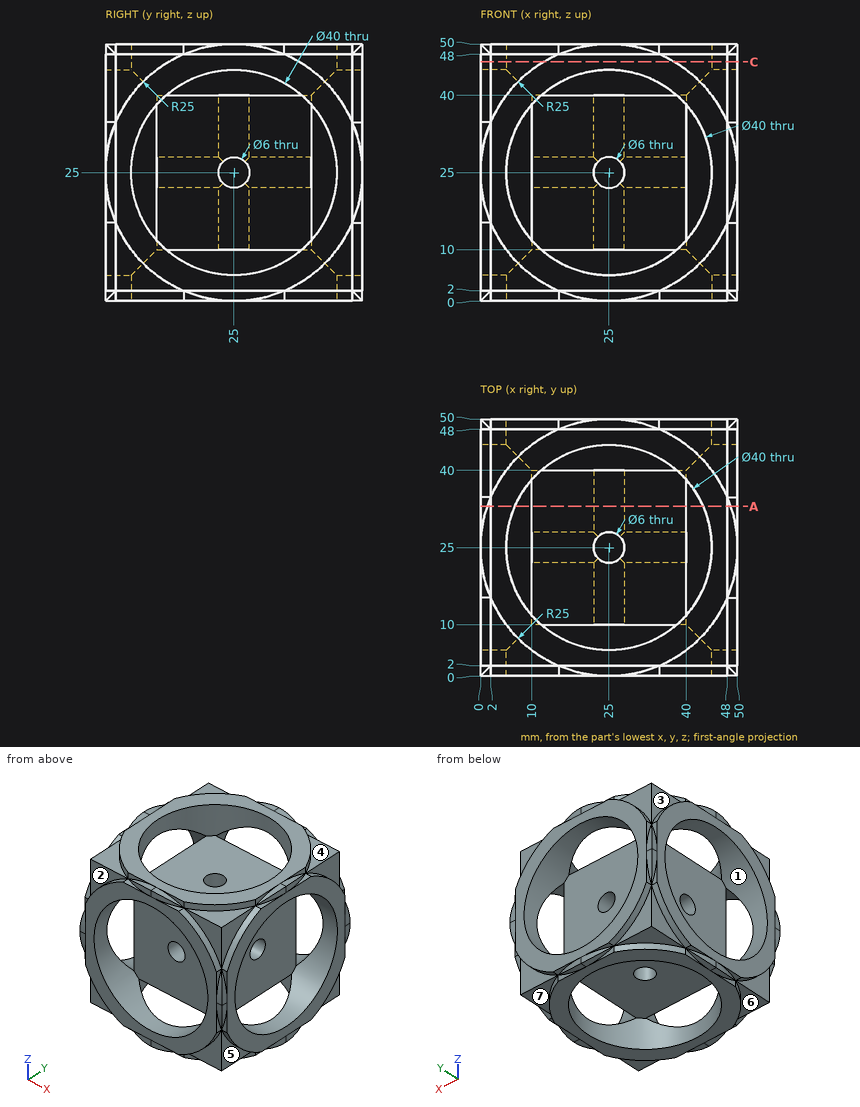
Design review of the part shown in the three views and the two pictorial views. Dimensions are in mm from the part's minimum x, y and z. A direction names the side the tool comes from. Round coordinates to 2 decimals unless told otherwise and drop trailing zeros. Write each loop counter-clockwise with the first axis right and the second up, starting at its lowest first coordinate (ties: lowest second). Pieces come first, ordered by that corner, then holes. Notation, with made-up numbers: (69.25, -9) - (83.25, -9) arc R17 cw to (83.25, 24) - close; hole circle Ø8 at (67, 25.25). An arc over 180 degrees is marked (long way). Write item = value, one per line. Start each with the question number.
1. Consider section C-C on z = 46.5. State the section outline as (x, y) points, plus the area to 3 significant figures.
2. Draft analysis for pull direction Y (two halves, no side actions). For the marked faces 1, 2 and 3, state which applies: released by +Y, released by -Y, zero draft, split by the parting line, or undercut.
3. For the marked faces 4, 5, 6 and 7, list the 3-axis set-ups (+Z, -Z, +X, -X, +Y, -Y) from which the entire face can be reached by the end or side of a thin tool; tool diameter is ignored.
4. Wall thickness on L1, parallel to Z at x = 33, y = 36; L2, parallel to Z at x = 17.5, y = 44: over which ranges is each line inside the solid? List them lowest first.
5. For pin 1 Ø24 at (y, z) = (25, 31.5) entering from -X; pin 2 Ø12 at (x, y) = (17, 22.5) entering from -Z; pin 3 Ø3 at (x, z) = (31, 23) entering from -Y, all flat-tipped, find the tip position at first contact; note any pin that passes through.
6. Consider section A-A on y = 33. Give the number of separate pieces and of enclosed holes in the cut face, plus the area to 3 significant figures.
Evaluation:
q1.outline = (0, 12.24) - (2, 12.24) - (2, 2) - (12.24, 2) - (12.24, 0) - (37.76, 0) - (37.76, 2) - (48, 2) - (48, 12.24) - (50, 12.24) - (50, 37.76) - (48, 37.76) - (48, 48) - (37.76, 48) - (37.76, 50) - (12.24, 50) - (12.24, 48) - (2, 48) - (2, 37.76) - (0, 37.76) - close; hole circle Ø40 at (25, 25)
q1.area = 1,060 mm2
q2.face_1 = undercut
q2.face_2 = released by -Y
q2.face_3 = zero draft
q3.face_4 = +Z, +X, +Y
q3.face_5 = -Z, +X, -Y
q3.face_6 = -Z, -X, -Y
q3.face_7 = -Z, +X, +Y
q4.L1 = 10 to 40
q4.L2 = 0 to 6.46, 43.54 to 50
q5.pin_1 = 10
q5.pin_2 = 10
q5.pin_3 = 10
q6.separate_pieces = 5
q6.enclosed_holes = 1
q6.area = 1,040 mm2
